Read the model definition and answer for the solid it produces. Units are mm, in the model's axes. Face numbers are marked on the shaded views. A direction names the side the tool comes from. Round coordinates to 2 decimals unless told otherwise and drop trailing zeros. Loops run counter-clockwise (first coordinate to the right, second up) from the corner with the lowest first, then second, coordinate; pieces in that order, holes last. Notation, with made-up numbers: (-30, 87) - (29, 87) arc R20 ccw to (29, 111) - close; hole circle Ø11 at (-14.75, 2). An arc over 180 degrees is marked (long way). Answer as CSV lines item,"result".
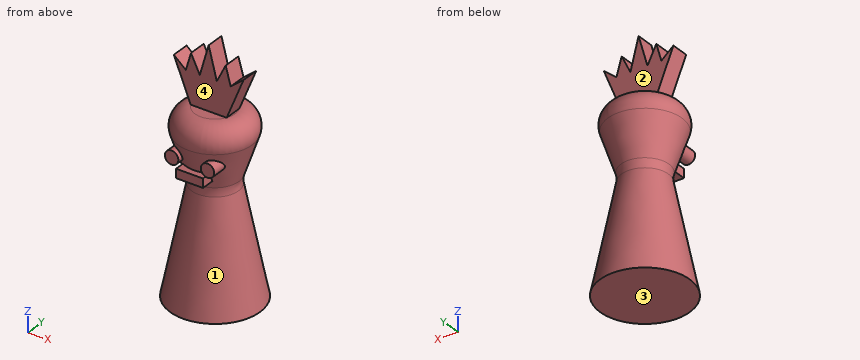
```python
from build123d import *

# Parameters (mm, degrees)
F2_R     = 5.08
F4_DEPTH = 2.54
F5_R     = 1.905
F5_W     = 7.62
F5_H     = 2.54
F6_DEPTH = 10.16


with BuildPart() as f1:
    # F0 (on Front) → F1 (revolve)
    with BuildSketch(Plane.XZ):
        Polygon((12.7, 50.8), (12.7, 0), (25.4, 0), (19.05, 31.75), (25.4, 50.8), align=None)
    revolve(axis=Axis((12.7, 0, 25.4), (0, 0, -1)))

    # F2
    f2_edges = [f1.edges().sort_by_distance(p)[0] for p in [
        (0, 0, 50.8),
        (6.35, 0, 31.75),
    ]]
    fillet(f2_edges, radius=F2_R)

    # F3 (on Front) → F4 (join, symmetric)
    with BuildSketch(Plane.XZ):
        Polygon((2.8545528618, 62.5720224929), (7.62, 50.8), (17.78, 50.8), (22.5454471382, 62.5720224929), (18.9388975427, 59.6384511692), (17.489523992, 64.7184511692), (15.004631497, 59.6384511692), (12.7, 68.5284511692), (10.187403664, 59.6384511692), (7.702511169, 64.7184511692), (6.2521615923, 59.6384511692), align=None)
    extrude(amount=F4_DEPTH, both=True)

    # F5 (on Front) → F6 (join)
    with BuildSketch(Plane.XZ):
        with Locations((7.62, 40.3035629486)):
            Circle(F5_R)
        with Locations((17.78, 40.3035629486)):
            Circle(F5_R)
        with Locations((12.7, 36.4935629486)):
            Rectangle(F5_W, F5_H)
    extrude(amount=F6_DEPTH)


solid = f1.part
```
1) Find the intervals of material crossed by line 1 (Y direction, x = 12, z = 56); line 2 (Z direction, x = 16.75, y = 3); line 3 (Y direction, x = 14.25, z = 36), in increasing order.
Entries:
line 1,"y = -2.54 to 2.54"
line 2,"z = 0 to 50.8"
line 3,"y = -10.16 to 7.61"
2) A cutting plane is placed at A-A, the plane z = 60.5. Determine the outline of the cut face in (x, y).
Entries:
outline,"(3.69, -2.54) - (5.25, -2.54) - (5.25, 2.54) - (3.69, 2.54) - close; (6.5, -2.54) - (9.77, -2.54) - (9.77, 2.54) - (6.5, 2.54) - close; (10.43, -2.54) - (14.78, -2.54) - (14.78, 2.54) - (10.43, 2.54) - close; (15.43, -2.54) - (18.69, -2.54) - (18.69, 2.54) - (15.43, 2.54) - close; (20, -2.54) - (21.71, -2.54) - (21.71, 2.54) - (20, 2.54) - close"
3) A tool of negligible diameter and unlimited length cuts with its end or side. For the marked faces 1, 2, 3 and 4, from which of +Z, -Z, +X, -X, +Y, -Y can it reach the whole face along a straight path? Write none if from no direction.
Entries:
face 1,"none"
face 2,"+Z, +X, -X, +Y"
face 3,"-Z, +X, -X, +Y, -Y"
face 4,"+Z, +X, -X, -Y"
4) Each of these flat-tipped pins is pushed along its axis until it touches: P1, Ø1.6, axis at x = 13, y = -4, coming from the +Z side; P2, Ø9, axis at x = 17.5, z = 57.5, coming from the +Y side; P3, Ø3, axis at x = 17.5, z = 40.5, coming from the -Y side. Where does it stop, or does it pass through?
Entries:
P1,"stops at z = 50.8"
P2,"stops at y = 2.54"
P3,"stops at y = -10.16"
5) A cutting plane is placed at B-B, the plane z = 25.5. Determine the outline of the cut face in (x, y), plus the area to 3 significant figures.
Entries:
outline,"circle Ø15.2 at (12.7, 0)"
area,"181 mm^2"
6) A cutting plane is placed at C-C, the plane x = 20.75. Count the separate pieces of the cut face and the enclosed holes in it, plus the area to 3 significant figures.
Entries:
separate pieces,"3"
enclosed holes,"0"
area,"442 mm^2"
